from build123d import *

# Parameters (mm, degrees)
SKETCH1_W           = 10
SKETCH1_H           = 143
SKETCH1_R           = 3
BOSS_EXTRUDE1_DEPTH = 6
CHAMFER1_SIZE       = 0.5


with BuildPart() as part:
    # Sketch1 → Boss-Extrude1 (new body)
    with BuildSketch(Plane.XY):
        Rectangle(SKETCH1_W, SKETCH1_H)
        with Locations((0, -56.5)):
            Circle(SKETCH1_R, mode=Mode.SUBTRACT)
        with Locations((0, -35.5)):
            Circle(SKETCH1_R, mode=Mode.SUBTRACT)
        with Locations((0, -8.5)):
            Circle(SKETCH1_R, mode=Mode.SUBTRACT)
        with Locations((0, 23.5)):
            Circle(SKETCH1_R, mode=Mode.SUBTRACT)
        with Locations((0, 61.5)):
            Circle(SKETCH1_R, mode=Mode.SUBTRACT)
        with Locations((0, 43.004767178)):
            Circle(SKETCH1_R, mode=Mode.SUBTRACT)
        with Locations((0, 7.137747133)):
            Circle(SKETCH1_R, mode=Mode.SUBTRACT)
        with Locations((0, -22.793294966)):
            Circle(SKETCH1_R, mode=Mode.SUBTRACT)
    extrude(amount=BOSS_EXTRUDE1_DEPTH)

    # Chamfer1
    chamfer1_edges = [part.edges().sort_by_distance(p)[0] for p in [
        (-3, -56.5, 6),
        (-3, -35.5, 6),
        (-3, -8.5, 6),
        (-3, 23.5, 6),
        (-3, 61.5, 6),
    ]]
    chamfer(chamfer1_edges, length=CHAMFER1_SIZE)


solid = part.part
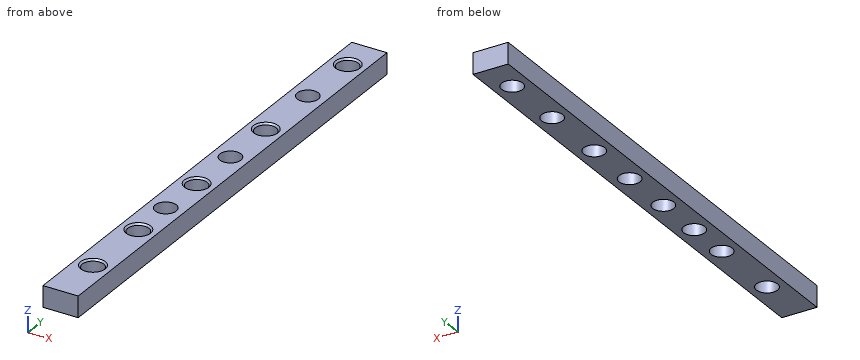
Read the model definition and answer for the solid it produces. Units are mm, in the model's axes. Round coordinates to 2 decimals unless told otherwise and drop trailing zeros. Order: outer loops, then holes, each group sorted by start corner. A loop starts at its lowest first (then second) coordinate and runs counter-clockwise, first axis right, second up.
1) The part is cut by section A-A on y = -56.5. Write down the section's boundary in (x, z).
2) The part is cut by section B-B on x = 0. Give the number of separate pieces and of enclosed holes in the cut face, plus the area to 3 significant figures.
3) A flat-ended cylindrical pin translates along its axis: pin 1 (2 mm diameter, centred on x = 2.5, y = 0, fed in from -Z). Find the tip coordinate at first contact, or state that the pin passes through.
4) A straight line is drawn through the part: L1, parallel to X at y = -34, z = 3.4. Find the intervals that lie inside material, in ascending order.
Resolved:
1. outline: (-5, 0) - (-3, 0) - (-3, 5.5) - (-3.5, 6) - (-5, 6) - close; (3, 0) - (5, 0) - (5, 6) - (3.5, 6) - (3, 5.5) - close
2. separate pieces: 9
2. enclosed holes: 0
2. area: 569 mm2
3. pin 1: stops at z = 0
4. L1: x = -5 to -2.6, 2.6 to 5
